CAD build for the part. Positions are in the model's coordinates, mm. Coordinates: 2 decimals unless noted, no trailing zeros. Write each loop counter-clockwise with the first axis right and the second up, starting at its lowest first coordinate (ties: lowest second). Pieces come first, ordered by that corner, then holes. Notation, with made-up numbers: (-3, 56) - (6, 56) arc R13 cw to (6, 73) - close; hole circle Ø11 at (-11, 22.25). An arc over 180 degrees is marked (long way). Answer in a Markdown table with one row per item. Add a question column.
Q1. Band-saw the part on A-A (y = 2.3). List the corners of the cut face in (x, z) (1 decimal).
Q2. Drill centre lines: line 1 along Z through (x, y) = (-11.5, 1); line 2 along Z through (x, y) = (-22.5, 1.55); line 3 along X through (y, z) = (2.95, 66.5). Where is each one in solid material? Low to high. Write a range as from..to.
Q3. Pin check, flat tips, straight feed: pin 1 (1.1 mm diameter, centred on x = -10.5, y = 2, fed in from +Z); pin 2 (1.5 mm diameter, centred on x = -40, y = 1.5, fed in from -Z); pin 3 (1.5 mm diameter, centred on y = 1.5, z = -15, fed in from -X). Stop position of each tip, or through.
Q4. Band-saw the part on C-C (z = 1.5). List the corners of the cut face in (x, y), and give its area (3 significant figures).
Q5. Band-saw the part on B-B (x = -38). List the corners of the cut face in (y, z), and give its area (3 significant figures).
Autodesk Inventor part; units mm, degrees
ref_plane "YZ Plane" through (0, 0, 0) normal (1, 0, 0) x (0, 1, 0)
ref_plane "XZ Plane" through (0, 0, 0) normal (0, 1, 0) x (-1, 0, 0)
ref_plane "XY Plane" through (0, 0, 0) normal (0, 0, 1) x (1, 0, 0)
sketch "Sketch1" plane through (0, 0, 0) normal (0, 1, 0) x (-1, 0, 0)
  line L0 (9.0102, -12.8984) -> (9.0102, -15.8984)
  line L1 (9.0102, 95.1016) -> (9.0102, 98.1016)
  line L2 (9.0102, -15.8984) -> (-4.9898, -15.8984)
  line L3 (9.0102, 98.1016) -> (-4.9898, 98.1016)
  line L4 (-4.9898, 98.1016) -> (-4.9898, 95.1016)
  line L5 (-4.9898, 95.1016) -> (-7.9898, 95.1016)
  line L6 (-7.9898, 95.1016) -> (-7.9898, -12.8984)
  line L7 (-7.9898, -12.8984) -> (-4.9898, -12.8984)
  line L8 (-4.9898, -12.8984) -> (-4.9898, -15.8984)
  line L9 (9.0102, 95.1016) -> (11.1769, 95.1016)
  line L10 (11.1769, -12.8984) -> (9.0102, -12.8984)
  line L11 (82.0102, 18.2445) -> (82.0102, 63.9587)
  arc A0 (75.2535, 8.785) -> (82.0102, 18.2445) centre (72.0102, 18.2445) ccw
  arc A1 (82.0102, 63.9587) -> (75.2535, 73.4182) centre (72.0102, 63.9587) ccw
  line L12 (12.7985, -12.6281) -> (75.2535, 8.785)
  arc A2 (11.1769, -12.8984) -> (12.7985, -12.6281) centre (11.1769, -7.8984) ccw
  line L13 (12.7985, 94.8313) -> (75.2535, 73.4182)
  arc A3 (12.7985, 94.8313) -> (11.1769, 95.1016) centre (11.1769, 90.1016) ccw
  point P0 (0, 0)
extrude "Extrusion1" add sketch "Sketch1" along normal blind 3
properties part number "rearCover" material "Polycarbonate, Clear"
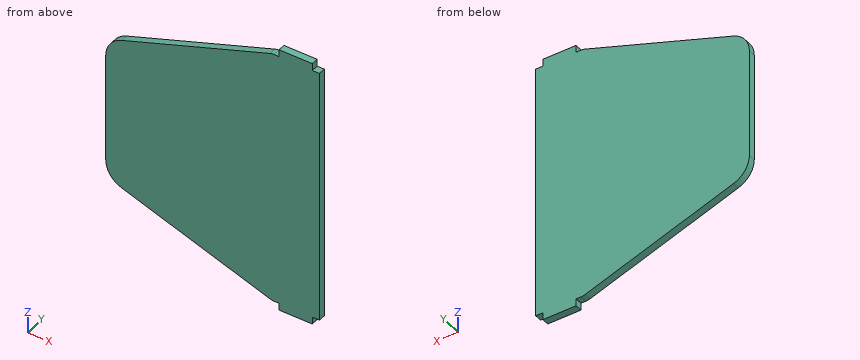
Checked values:
| question | item | result |
|---|---|---|
| 1 | outline | (-82, 18.2) arc R10 ccw to (-75.3, 8.8) - (-12.8, -12.6) arc R5 ccw to (-11.2, -12.9) - (-9, -12.9) - (-9, -15.9) - (5, -15.9) - (5, -12.9) - (8, -12.9) - (8, 95.1) - (5, 95.1) - (5, 98.1) - (-9, 98.1) - (-9, 95.1) - (-11.2, 95.1) arc R5 ccw to (-12.8, 94.8) - (-75.3, 73.4) arc R10 ccw to (-82, 64) - close |
| 2 | line 1 | z = -12.89..95.09 |
| 2 | line 2 | z = -9.3..91.51 |
| 2 | line 3 | x = -81.68..7.99 |
| 3 | pin 1 | stops at z = 95.1 |
| 3 | pin 2 | stops at z = -3.56 |
| 3 | pin 3 | stops at x = -9.01 |
| 4 | outline | (-54.01, 0) - (7.99, 0) - (7.99, 3) - (-54.01, 3) - close |
| 4 | area | 186 mm² |
| 5 | outline | (0, -3.99) - (3, -3.99) - (3, 86.19) - (0, 86.19) - close |
| 5 | area | 271 mm² |
